from build123d import *

# Parameters (mm, degrees)
F0_W     = 25.4
F0_H     = 50.8
F0_W_2   = 16.5
F0_H_2   = 19.372893
F1_DEPTH = 6.35
F2_R     = 1.815
F3_DEPTH = 3.302


with BuildPart() as f1:
    # F0 (on Top) → F1 (new body)
    with BuildSketch(Plane.XY):
        Rectangle(F0_W, F0_H)
        with Locations((-0.005, 10.513554)):
            Rectangle(F0_W_2, F0_H_2, mode=Mode.SUBTRACT)
    extrude(amount=F1_DEPTH)

    # F2 (on face) → F3 (join)
    with BuildSketch(Plane(origin=(0, 25.4, 0), x_dir=(-1, 0, 0), z_dir=(0, 1, 0))):
        with Locations((0, 3.175)):
            Circle(F2_R)
    extrude(amount=F3_DEPTH)


solid = f1.part
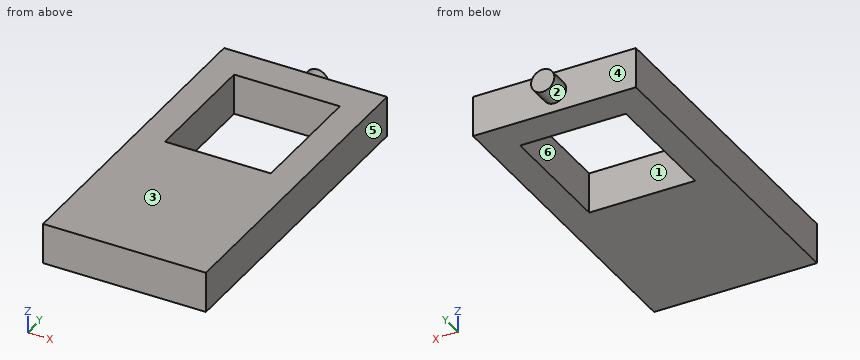
Check sheet for the modelled part. Datum: model origin and axes. Units: mm. Face numbers are marked on the shaded views. A direction names the side the tool comes from. Coordinates: 2 decimals unless noted, no trailing zeros. Write each loop counter-clockwise with the first axis right and the second up, starting at its lowest first coordinate (ties: lowest second). Pieces come first, ordered by that corner, then holes.
Item 1: Cross-section at C-C on y = 7. Record the boundary of the cut face in (x, z) (3 decimals).
Numbers:
outline: (-12.7, 0) - (-8.255, 0) - (-8.255, 6.35) - (-12.7, 6.35) - close; (8.245, 0) - (12.7, 0) - (12.7, 6.35) - (8.245, 6.35) - close
Item 2: Scan lines: probe 1 along Y at (x, z) = (3.5, 0.75); probe 2 along X at (y, z) = (11, 3) (3 decimals); probe 3 along Y at (x, z) = (-1.25, 2.25). Record each from-to range of solid material in increasing order.
Numbers:
probe 1: y = -25.4 to 0.83, 20.2 to 25.4
probe 2: x = -12.7 to -8.255, 8.245 to 12.7
probe 3: y = -25.4 to 0.83, 20.2 to 28.7
Item 3: Cross-section at A-A on x = 3. Record the boundary of the cut face in (y, z).
Numbers:
outline: (-25.4, 0) - (0.83, 0) - (0.83, 6.35) - (-25.4, 6.35) - close; (20.2, 0) - (25.4, 0) - (25.4, 6.35) - (20.2, 6.35) - close
Item 4: Access from +Z, -Z, +X, -X, +Y, -Y to the whole of each face (thin tool, end or side, straight path). Record for the marked faces 1, 2 and 3.
Numbers:
face 1: +Z, -Z
face 2: +Y
face 3: +Z, +X, -X, +Y, -Y
Item 5: Cross-section at B-B on z = 5.5. Record the boundary of the cut face in (x, y) (3 decimals).
Numbers:
outline: (-12.7, -25.4) - (12.7, -25.4) - (12.7, 25.4) - (-12.7, 25.4) - close; hole (-8.255, 0.827) - (8.245, 0.827) - (8.245, 20.2) - (-8.255, 20.2) - close
Item 6: Depth check by flat-ended pin: pin 1 Ø1 at (x, z) = (7.5, 3) entering from +Y. Enter the tip coordinate at first touch or a pass-through.
Numbers:
pin 1: stops at y = 25.4
Item 7: Cross-section at D-D on x = 0. Record the boundary of the cut face in (y, z), then the cut area to 3 significant figures.
Numbers:
outline: (-25.4, 0) - (0.83, 0) - (0.83, 6.35) - (-25.4, 6.35) - close; (20.2, 0) - (25.4, 0) - (25.4, 1.36) - (28.7, 1.36) - (28.7, 4.99) - (25.4, 4.99) - (25.4, 6.35) - (20.2, 6.35) - close
area: 212 mm2
Item 8: Mould release check, pull along X, two halves, no side actions. Record for the marked faces 4, 5 and 6: released by +X, released by -X, zero draft, split by the parting line, or undercut.
Numbers:
face 4: zero draft
face 5: released by +X
face 6: undercut
